Job drawing, mm, ordinate dimensions from the low corner. One solid piece. A direction names the side the tool comes from. Give positions to 0.01 mm unless a question says otherwise; leave off trailing zeros. Write each loop counter-clockwise with the first axis right and the second up, starting at its lowest first coordinate (ties: lowest second). Pieces come first, ordered by that corner, then holes. Notation, with made-up numbers: M 70.25,-39 L 108.25,-39 A11 ccw 108.25,-25 Z; hole C 35.5,43.25 d11. An arc over 180 degrees is marked long. Use a Markdown table: item, result.
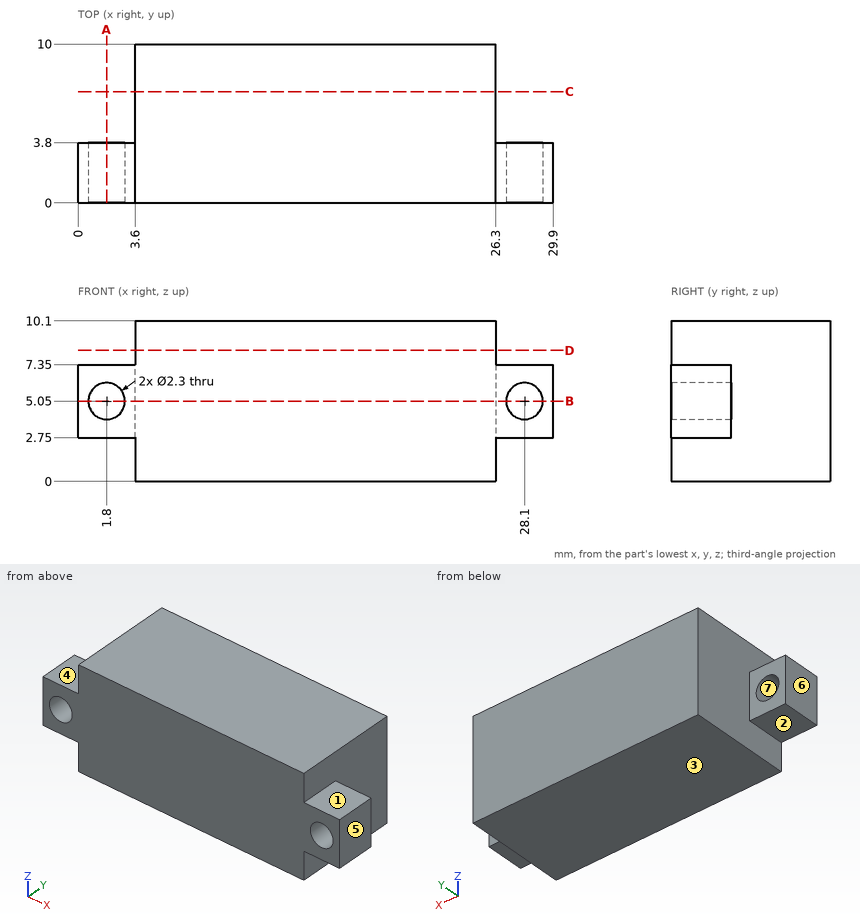
1. Cut at B-B, the plane z = 5.05. Give the cut face in (x, y), then the cut area to 3 significant figures.
Findings below:
| item | result |
|---|---|
| outline | M 0,0 L 0.65,0 L 0.65,3.8 L 0,3.8 Z; M 2.95,0 L 26.95,0 L 26.95,3.8 L 26.3,3.8 L 26.3,10 L 3.6,10 L 3.6,3.8 L 2.95,3.8 Z; M 29.25,0 L 29.9,0 L 29.9,3.8 L 29.25,3.8 Z |
| area | 237 mm2 |
2. Cut at C-C, the plane y = 7. Give the cut face in (x, z).
Findings below:
| item | result |
|---|---|
| outline | M 3.6,0 L 26.3,0 L 26.3,10.1 L 3.6,10.1 Z |
3. Cut at D-D, the plane z = 8.25. Give the cut face in (x, y), then the cut area to 3 significant figures.
Findings below:
| item | result |
|---|---|
| outline | M 3.6,0 L 26.3,0 L 26.3,10 L 3.6,10 Z |
| area | 227 mm2 |
4. Drop flat-ended pins along their axis: P1, Ø3, axis at x = 1.8, z = 5.05, coming from the -Y side; P2, Ø4, axis at x = 1.5, y = 2, coming from the +Z side; P3, Ø3, axis at y = 5.5, z = 6.5, coming from the -X side; P4, Ø2.5, axis at x = 28.1, z = 5.05, coming from the +Y side. Give the stop position or say it passes through.
Findings below:
| item | result |
|---|---|
| P1 | y = 0 |
| P2 | z = 7.35 |
| P3 | x = 3.6 |
| P4 | y = 3.8 |
5. Drill centre lines: L1, parallel to X at y = 2.75, z = 5.05; L2, parallel to X at y = 8.25, z = 4.25; L3, parallel to Z at x = 2.25, y = 2. Where is each one in solid material? Low to high.
Findings below:
| item | result |
|---|---|
| L1 | 0 to 0.65, 2.95 to 26.95, 29.25 to 29.9 |
| L2 | 3.6 to 26.3 |
| L3 | 2.75 to 3.99, 6.11 to 7.35 |
6. Cut at A-A, the plane x = 1.8. Give the cut face in (y, z).
Findings below:
| item | result |
|---|---|
| outline | M 0,2.75 L 3.8,2.75 L 3.8,3.9 L 0,3.9 Z; M 0,6.2 L 3.8,6.2 L 3.8,7.35 L 0,7.35 Z |
7. Tool access for the marked faces 1, 2 and 3: list every direction of +Z, -Z, +X, -X, +Y, -Y with a clear straight run to the whole face (end or side of a thin tool).
Findings below:
| item | result |
|---|---|
| face 1 | +Z, +X, +Y, -Y |
| face 2 | -Z, -X, +Y, -Y |
| face 3 | -Z, +X, -X, +Y, -Y |
8. Two-plate mould, pull along X, no slides. Class the marked faces 4, 5, 6 and 7: released by +X, released by -X, zero draft, split by the parting line, or undercut.
Findings below:
| item | result |
|---|---|
| face 4 | zero draft |
| face 5 | released by +X |
| face 6 | released by -X |
| face 7 | undercut |
